The figure shows three views and two pictorial views of one solid part (mm, origin at its lowest corner). Answer the questions. Coordinates: 2 decimals unless noted, no trailing zeros. Loops run counter-clockwise (first coordinate to the right, second up) from the corner with the lowest first, then second, coordinate; pieces in that order, holes last.
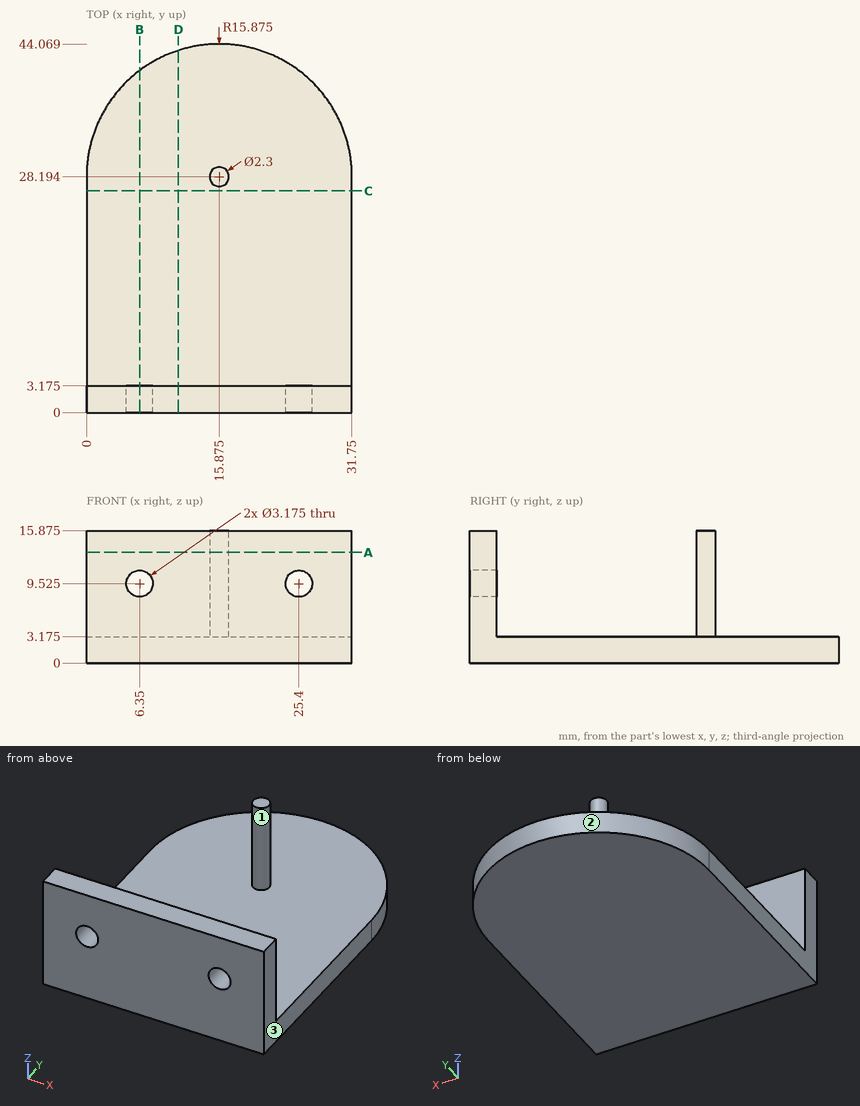
1. A cutting plane is placed at C-C, the plane y = 26.5. Give the vertices of the cut face in (x, z) (3 decimals).
2. A cutting plane is placed at B-B, the plane x = 6.35. Give the vertices of the cut face in (y, z) (1 decimal).
3. Each of these flat-tipped pins is pushed along its axis until it touches: P1, Ø3, axis at x = 25.4, z = 9.525, coming from the -Y side; P2, Ø1, axis at x = 16.5, z = 3.5, coming from the +Y side; P3, Ø4, axis at x = 22, y = 12, coming from the -Z side; P4, Ø5, axis at x = 6.5, z = 11, coming from the +Y side (3 decimals). Where does it stop, or does it pass through?
4. Determine the mould class of the marked faces 1, 2 and 3 for opening direction Y: released by +Y, released by -Y, zero draft, split by the parting line, or undercut.
5. Straight lines are drawn through the part: probe 1 along Z at (x, y) = (25.4, 1) (1 decimal); probe 2 along Z at (x, y) = (16.5, 20) (3 decimals). For each, find the intervals that lie inside material, in ascending order.
6. A cutting plane is placed at D-D, the plane x = 11. Give the vertices of the cut face in (y, z) (3 decimals), then the cut area to 3 significant figures.
7. A cutting plane is placed at A-A, the plane z = 13.25. Give the vertices of the cut face in (x, y) (3 decimals), then the cut area to 3 significant figures.
Answers below:
1. outline: (0, 0) - (31.75, 0) - (31.75, 3.175) - (0, 3.175) - close
2. outline: (0, 0) - (40.9, 0) - (40.9, 3.2) - (3.2, 3.2) - (3.2, 7.9) - (0, 7.9) - close; (0, 11.1) - (3.2, 11.1) - (3.2, 15.9) - (0, 15.9) - close
3. P1: passes through
3. P2: stops at y = 44.07
3. P3: stops at z = 0
3. P4: stops at y = 3.175
4. face 1: undercut
4. face 2: released by +Y
4. face 3: zero draft
5. probe 1: z = 0 to 7.9, 11.1 to 15.9
5. probe 2: z = 0 to 3.175
6. outline: (0, 0) - (43.302, 0) - (43.302, 3.175) - (3.175, 3.175) - (3.175, 15.875) - (0, 15.875) - close
6. area: 178 mm2
7. outline: (0, 0) - (31.75, 0) - (31.75, 3.175) - (0, 3.175) - close; circle Ø2.3 at (15.875, 28.194)
7. area: 105 mm2
